```python
from build123d import *

# Parameters (mm, degrees)
SKETCH1_W                = 18
SKETCH1_H                = 64
BOSS_EXTRUDE1_DEPTH      = 6.35
M3_CLEARANCE_HOLE1_D     = 3.2
M3_CLEARANCE_HOLE1_DEPTH = 7.5
M3_CLEARANCE_HOLE1_TIP   = 0.96137699
SKETCH4_W                = 10
SKETCH4_H                = 37.5
CUT_EXTRUDE1_DEPTH       = 7.35
FILLET1_R                = 3


with BuildPart() as part:
    # Sketch1 → Boss-Extrude1 (new body)
    with BuildSketch(Plane.XY):
        Rectangle(SKETCH1_W, SKETCH1_H)
    extrude(amount=BOSS_EXTRUDE1_DEPTH)

    # M3 Clearance Hole1
    with Locations(Plane(origin=(-4, 15, 6.35), x_dir=(1, 0, 0), z_dir=(0, 0, 1))):
        with Locations((0, 0), (0, 13), (8, 13), (8, 0)):
            Hole(M3_CLEARANCE_HOLE1_D / 2, depth=M3_CLEARANCE_HOLE1_DEPTH)
            with Locations((0, 0, -(M3_CLEARANCE_HOLE1_DEPTH + M3_CLEARANCE_HOLE1_TIP / 2))):  # 118° drill point
                Cone(0, M3_CLEARANCE_HOLE1_D / 2, M3_CLEARANCE_HOLE1_TIP, mode=Mode.SUBTRACT)

    # Sketch4 → Cut-Extrude1 (cut, through all)
    with BuildSketch(Plane.XY.offset(6.35)):
        with Locations((0, -9.25)):
            Rectangle(SKETCH4_W, SKETCH4_H)
    extrude(amount=-CUT_EXTRUDE1_DEPTH, mode=Mode.SUBTRACT)

    # Fillet1
    fillet1_edges = [part.edges().sort_by_distance(p)[0] for p in [
        (5, -9.25, 6.35),
        (0, 9.5, 6.35),
        (-5, -9.25, 6.35),
        (0, -28, 6.35),
    ]]
    fillet(fillet1_edges, radius=FILLET1_R)


solid = part.part
```
The model under review builds one solid part; all positions refer to its coordinate system, in mm. A direction names the side the tool comes from. Round coordinates to 2 decimals unless told otherwise and drop trailing zeros. Order: outer loops, then holes, each group sorted by start corner. A loop starts at its lowest first (then second) coordinate and runs counter-clockwise, first axis right, second up. Notation, with made-up numbers: (73.5, -5) -> (115.5, -5) arc R10 ccw to (115.5, 8) -> close; hole circle Ø5 at (61.25, -16.75). An arc over 180 degrees is marked (long way). One line per item, written item: value. Start each with the question number.
Q1. Take a section at A-A (x = -4). Write out the cut boundary in (y, z).
Q2. Wall thickness on line 1 (Y direction, x = -4, z = 1.5); line 2 (X direction, y = -13.5, z = 3); line 3 (Y direction, x = -2, z = 3.25): over which ranges is each line inside the solid? List them lowest first.
Q3. Mouldability with a two-part tool opening along Y and no side actions: class faces 4 (the face through (0, 32, 3)), 5 (the face through (0, -32, 3)), 6 (the face through (9, 0, 3)), 7 (the face through (4.208, 29.586, 3.131)) as released by +Y, released by -Y, zero draft, split by the parting line, or undercut.
Q4. Take a section at C-C (y = 28). Write out the cut boundary in (x, z), and give its area (3 significant figures).
Q5. Take a section at D-D (x = 1.5). Write out the cut boundary in (y, z).
Q6. Take a section at B-B (z = 2.5). Write out the cut boundary in (x, y).
Q7. Machinability: for faces 1 (the face through (0, -28, 2)), 2 (the face through (5.9, -8.95, 5.49)), 3 (the face through (-6, 8, 0)), which of the approach directions +Z, -Z, +X, -X, +Y, -Y give a long, thin tool a straight path to every point of the face, cutting with its end or side? Answer none if there is none.
Q8. Clearance check with a flat-ended pin moving along its axis: pin 1 Ø3 at (x, y) = (4, 11) entering from +Z. State where the tip first meets the part, or that it passes through.
Reported:
1. outline: (-32, 0) -> (-28, 0) -> (-28, 3.35) arc R3 ccw to (-31, 6.35) -> (-32, 6.35) -> close; (9.5, 0) -> (13.4, 0) -> (13.4, 6.35) -> (12.5, 6.35) arc R3 ccw to (9.5, 3.35) -> close; (16.6, 0) -> (26.4, 0) -> (26.4, 6.35) -> (16.6, 6.35) -> close; (29.6, 0) -> (32, 0) -> (32, 6.35) -> (29.6, 6.35) -> close
2. line 1: y = -32 to -28, 9.5 to 13.4, 16.6 to 26.4, 29.6 to 32
2. line 2: x = -9 to -5, 5 to 9
2. line 3: y = -32 to -28, 9.5 to 32
3. face 4: released by +Y
3. face 5: released by -Y
3. face 6: zero draft
3. face 7: undercut
4. outline: (-9, 0) -> (-5.6, 0) -> (-5.6, 6.35) -> (-9, 6.35) -> close; (-2.4, 0) -> (2.4, 0) -> (2.4, 6.35) -> (-2.4, 6.35) -> close; (5.6, 0) -> (9, 0) -> (9, 6.35) -> (5.6, 6.35) -> close
4. area: 73.7 mm2
5. outline: (-32, 0) -> (-28, 0) -> (-28, 3.35) arc R3 ccw to (-31, 6.35) -> (-32, 6.35) -> close; (9.5, 0) -> (32, 0) -> (32, 6.35) -> (12.5, 6.35) arc R3 ccw to (9.5, 3.35) -> close
6. outline: (-9, -32) -> (9, -32) -> (9, 32) -> (-9, 32) -> close; hole circle Ø3.2 at (-4, 15); hole circle Ø3.2 at (-4, 28); hole (-5, -28) -> (5, -28) -> (5, 9.5) -> (-5, 9.5) -> close; hole circle Ø3.2 at (4, 15); hole circle Ø3.2 at (4, 28)
7. face 1: +Z, -Z
7. face 2: +Z
7. face 3: -Z, +X, -X, +Y, -Y
8. pin 1: stops at z = 6.35
